Input: part model. Units: mm. Frame: model coordinates. A direction names the side the tool comes from. Give positions to 0.01 mm unless a question says otherwise; leave off trailing zeros. Loops run counter-clockwise (first coordinate to the right, second up) from the corner with the lowest first, then second, coordinate; pieces in that order, holes last. Notation, with made-up numbers: M 21.5,-31.75 L 68.5,-31.75 A24 ccw 68.5,-2.75 Z; hole C 42,81.25 d1. An arc over 180 degrees is marked long. One line per item, written item: value. Start each with the question number.
(1) Section B-B on z = 5.25. Output: boundary loops of the cut face in (x, y), plus the area to 3 significant figures.
(2) Pin query (flat end, axial travel): P1, Ø19, axis at x = 124, y = -35, coming from the -Z side; P2, Ø1.2, axis at y = -41.5, z = -1.5, coming from the +X side; P3, Ø2, axis at x = 56, z = -2, coming from the +Y side; P4, Ø1.2, axis at y = -51, z = -2.5, coming from the -X side. Return the tip coordinate at first contact, or that it passes through.
(3) Section C-C on x = 71. Output: boundary loops of the cut face in (y, z).
(4) Section D-D on y = -63.5. Output: boundary loops of the cut face in (x, z), plus the area to 3 significant figures.
(5) Ray query, line 1 along X through (y, z) = (-66, 3.5); line 2 along X through (y, z) = (-67.5, 4.5); line 3 along Y through (x, z) = (121, 0.5). Return the intervals inside material, ascending. Write a range as from..to.
(6) Access query for faces 4 (the cylindrical face through (131.23, -3.99, 6.08)), 5 (the flat face through (19, -40, 0)), 6 (the flat face through (68, -40, 8.946)). Directions: +Z, -Z, +X, -X, +Y, -Y. A direction counts if a zero-diameter tool reaches every point of the face in a straight line with its end or side. Return the directions, or none.
(7) Pull-direction query (X, two-part tool) for faces 1 (the flat face through (97.443, -40, -2)), 2 (the flat face through (116, -40, 0)), 3 (the cylindrical face through (9.802, -69.155, 5.916)); classes: released by +X, released by -X, zero draft, split by the parting line, or undercut.
(8) Section A-A on y = -21.5. Output: boundary loops of the cut face in (x, z).
```python
from build123d import *

# Parameters (mm, degrees)
F1_DEPTH = 82
F2_R     = 5.5
F3_DEPTH = 12.001
F4_R     = 14


with BuildPart() as f1:
    # F0 (on Front) → F1 (new body)
    with BuildSketch(Plane.XZ):
        with BuildLine():
            Line((0, 12), (0, 0))
            Line((0, 0), (38, 0))
            Line((38, 0), (38, -4))
            Line((38, -4), (97.442689, -4))
            Line((97.442689, -4), (97.442689, 0))
            Line((97.442689, 0), (135.442689, 0))
            Line((135.442689, 0), (135.442689, 12))
            Line((135.442689, 12), (91.442689, 12))
            Line((91.442689, 12), (91.442689, 11.946312))
            ThreePointArc((91.442689, 11.946312), (90.56401, 9.824992), (88.442689, 8.946312))
            Line((88.442689, 8.946312), (47.000647, 8.946312))
            ThreePointArc((47.000647, 8.946312), (44.889444, 9.814922), (44.000783, 11.917763))
            Line((44.000783, 11.917763), (44, 12))
            Line((44, 12), (0, 12))
        make_face()
    extrude(amount=F1_DEPTH)

    # F2 (on Top) → F3 (cut, through all)
    with BuildSketch(Plane.XY):
        with Locations((12.620713, -11.808709)):
            Circle(F2_R)
        with Locations((120.620713, -11.808709)):
            Circle(F2_R)
        with Locations((14.166683, -65.808709)):
            Circle(F2_R)
        with Locations((122.166683, -65.808709)):
            Circle(F2_R)
    extrude(amount=F3_DEPTH, mode=Mode.SUBTRACT)

    # F4
    f4_edges = [f1.edges().sort_by_distance(p)[0] for p in [
        (135.442689, 0, 6),
        (135.442689, -82, 6),
        (0, -82, 6),
        (0, 0, 6),
    ]]
    fillet(f4_edges, radius=F4_R)


solid = f1.part
```
Output values:
1. outline: M 0,-68 A14 ccw 14,-82 L 121.44,-82 A14 ccw 135.44,-68 L 135.44,-14 A14 ccw 121.44,0 L 14,0 A14 ccw 0,-14 Z; hole C 12.62,-11.81 d11; hole C 14.17,-65.81 d11; hole C 120.62,-11.81 d11; hole C 122.17,-65.81 d11
1. area: 10,600 mm²
2. P1: stops at z = 0
2. P2: stops at x = 97.44
2. P3: stops at y = 0
2. P4: stops at x = 38
3. outline: M -82,-4 L 0,-4 L 0,8.95 L -82,8.95 Z
4. outline: M 0,0 L 9.17,0 L 9.17,12 L 0,12 Z; M 19.16,0 L 38,0 L 38,-4 L 97.44,-4 L 97.44,0 L 117.17,0 L 117.17,12 L 91.44,12 L 91.44,11.95 A3 cw 88.44,8.95 L 47,8.95 A3 cw 44,11.92 L 44,12 L 19.16,12 Z; M 127.16,0 L 135.44,0 L 135.44,12 L 127.16,12 Z
4. area: 1,480 mm²
5. line 1: x = 0..8.67, 19.66..116.67, 127.66..135.44
5. line 2: x = 0..8.93, 19.4..116.93, 127.4..135.44
5. line 3: y = -82..-71.18, -60.43..-17.3, -6.32..0
6. face 4: +Z, -Z, +X, +Y
6. face 5: -Z, -X, +Y, -Y
6. face 6: +Z, +Y, -Y
7. face 1: released by +X
7. face 2: zero draft
7. face 3: undercut
8. outline: M 0,0 L 38,0 L 38,-4 L 97.44,-4 L 97.44,0 L 135.44,0 L 135.44,12 L 91.44,12 L 91.44,11.95 A3 cw 88.44,8.95 L 47,8.95 A3 cw 44,11.92 L 44,12 L 0,12 Z
